Autodesk Inventor part; units mm, degrees
ref_plane "YZ Plane" through (0, 0, 0) normal (1, 0, 0) x (0, 1, 0)
ref_plane "XZ Plane" through (0, 0, 0) normal (0, 1, 0) x (-1, 0, 0)
ref_plane "XY Plane" through (0, 0, 0) normal (0, 0, 1) x (1, 0, 0)
sketch "Sketch1" plane through (0, 0, 0) normal (1, 0, 0) x (0, 1, 0)
  line L0 (0, 0) -> (15.2005, 26.3281)
  line L1 (15.2005, 26.3281) -> (43.7967, 9.8181)
  line L2 (0, -98.8011) -> (0, 41.6267)
  line L3 (43.7967, 9.8181) -> (0, -66.04)
  line L4 (0, 0) -> (0, -66.04)
  line L5 (19.05, 24.1056) -> (0, -8.89) construction
  dimension "d0" = 33.02
  dimension "d1" = 30
  dimension "d5" = 4.445
  dimension "d6" = 38.1
extrude "Extrusion1" add sketch "Sketch1" along normal mid plane 33.02
sketch "Sketch2" plane through (-16.51, 15.2005, 26.3281) normal (0, 0.5, 0.8660254) x (1, 0, 0)
  line L0 (0, 0) -> (33.02, 0) construction
  line L1 (33.02, 0) -> (33.02, 33.02) construction
  line L2 (0, 0) -> (33.02, 33.02) construction
  line L3 (33.02, 33.02) -> (0, 33.02) construction
  line L4 (0, 33.02) -> (33.02, 0) construction
  line L5 (3.175, 3.175) -> (29.845, 3.175)
  line L6 (29.845, 3.175) -> (29.845, 29.845)
  line L7 (29.845, 29.845) -> (3.175, 29.845)
  line L8 (3.175, 29.845) -> (3.175, 3.175)
  line L9 (3.175, 3.175) -> (29.845, 29.845) construction
  line L10 (29.845, 3.175) -> (3.175, 29.845) construction
  point P0 (16.51, 0)
  point P1 (16.51, 16.51)
  dimension "d7" = 26.67
extrude "Extrusion2" cut sketch "Sketch2" against normal blind 38.1
sketch "Sketch3" plane through (0, 0, 0) normal (1, 0, 0) x (0, 1, 0)
  line L0 (15.2005, 26.3281) -> (0, 0)
  line L1 (0, 0) -> (0, -66.04)
  line L2 (0, -66.04) -> (43.7967, 9.8181)
  line L3 (21.997, -21.59) -> (0, -8.89)
  line L4 (17.9501, 24.7406) -> (0, -6.35)
  line L5 (0, 0) -> (0, -66.04)
  line L6 (15.2005, 26.3281) -> (1.6498, 26.3281) construction
  line L7 (0, 0) -> (15.2005, 26.3281)
  line L8 (0, 0) -> (0, 51.7281)
  line L9 (43.7967, 9.8181) -> (0, -66.04)
  line L10 (0, -66.04) -> (0, -91.44)
  line L11 (0, -134.3611) -> (0, 77.1867)
  line L12 (0, 51.7281) -> (-3.175, 51.7281)
  line L13 (-3.175, 51.7281) -> (-3.175, -91.44)
  line L14 (-3.175, -91.44) -> (0, -91.44)
  point P0 (1.0999, -13.335)
  point P1 (0, -15.24)
  point P2 (0, -6.35)
  dimension "d10" = 25.4
  dimension "d11" = 25.4
  dimension "d12" = 3.175
  dimension "supportBaseLength" = 143.1681
extrude "Extrusion3" add sketch "Sketch3" along normal mid plane 22.86
sketch "Sketch5" plane through (0, 0, 0) normal (1, 0, 0) x (0, 1, 0)
  line L0 (0, 0) -> (15.2005, 26.3281)
  line L1 (0, 51.7281) -> (0, 0)
  line L2 (15.2005, 26.3281) -> (43.7967, 9.8181)
  line L3 (15.2005, 26.3281) -> (0, 26.3281)
  line L4 (0, 0) -> (15.2005, 26.3281)
extrude "Extrusion5" add sketch "Sketch5" along normal mid plane 22.86
sketch "Sketch4" plane through (0, 0, 0) normal (0, 0, 1) x (1, 0, 0)
  line L0 (16.51, 43.7967) -> (-16.51, 43.7967)
  line L1 (16.51, 0) -> (16.51, 43.7967)
  line L2 (16.51, 0) -> (11.43, 0)
  line L3 (11.43, 0) -> (-11.43, 0)
  line L4 (-11.43, 0) -> (-16.51, 0)
  line L5 (-16.51, 43.7967) -> (-16.51, 0)
  line L6 (-11.43, 0) -> (-11.43, -3.175)
  line L7 (11.43, -3.175) -> (-11.43, -3.175)
  line L8 (11.43, -3.175) -> (11.43, 0)
  line L9 (-11.43, 0) -> (-16.51, 5.08)
  line L10 (-16.51, 43.7967) -> (-16.51, 0)
  line L11 (-16.51, 5.08) -> (-16.51, 0)
  line L12 (0, 0) -> (0, 43.7967) construction
  line L13 (11.43, 0) -> (16.51, 0)
  line L14 (11.43, 0) -> (16.51, 5.08)
  line L15 (16.51, 5.08) -> (16.51, 0)
  dimension "d15" = 45
extrude "Extrusion4" cut sketch "Sketch4" against normal up to surface (143.1681 mm away) from surface at 51.7281 contours L1 L2 L14 | L9 L4 L5
sketch "Sketch6" plane through (-11.43, 0, 51.7281) normal (0, 1, 0) x (1, 0, 0)
  line L0 (22.86, 143.1681) -> (0, 143.1681) construction
  line L1 (11.43, 143.1681) -> (11.43, 0) construction
  line L2 (22.86, 0) -> (0, 0) construction
  point P0 (11.43, 51.7281)
  point P1 (11.43, 130.4681)
  point P2 (11.43, 12.7)
  dimension "d21" = 12.7
  dimension "d22" = 12.7
hole "Hole1" at (0, 0, -78.74) at (0, 0, 39.0281) direction (0, -1, 0) diameter 5.6134 end through all
sketch "Sketch9" plane through (0, 0, 0) normal (1, 0, 0) x (0, 1, 0)
  line L0 (1.905, -3.0504) -> (1.905, -9.9899)
  line L1 (1.905, -9.9899) -> (21.997, -21.59)
  line L2 (41.047, 11.4056) -> (21.997, -21.59)
  line L3 (17.9501, 24.7406) -> (41.047, 11.4056)
  line L4 (17.9501, 24.7406) -> (1.905, -3.0504)
  line L5 (29.4986, 18.0731) -> (10.4486, -14.9225) construction
  line L6 (1.905, -9.9899) -> (21.997, -21.59) construction
  circle A0 centre (19.9736, 1.5753) radius 2.8067
  point P0 (0, 0)
  dimension "d30" = 5.6134
extrude "Extrusion6" cut sketch "Sketch9" along normal through all both and the other way through all contours A0
sketch "Sketch10" plane through (-16.51, 43.7967, 9.8181) normal (0, 0.8660254, -0.5) x (1, 0, 0)
  line L0 (3.175, 0) -> (29.845, 0) construction
  line L1 (16.51, 0) -> (16.51, 77.7875) construction
  point P0 (16.51, 30.401)
  point P1 (16.51, 19.05)
  dimension "d33" = 19.05
hole "Hole2" at (0, 34.2717, -6.6797) direction (0, -0.8660254, 0.5) diameter 5.6134 depth 3.175
equation "\"d0\" = widthToSupportExtrusion"
equation "\"d1\" = attachementAngle"
equation "\"d6\" = insertDepth"
equation "\"d2\" = widthToSupportExtrusion"
equation "\"d7\" = insertForExtrusion"
equation "\"d8\" = insertDepth"
equation "\"d12\" = supportBaseDepth"
equation "\"d13\" = supportBaseWidth"
equation "\"attachementAngle\" = 30deg"
equation "\"extrusionSize\" = 25.4"
equation "\"wallThickness\" = 3.175"
equation "\"slipClearance\" = 0.635"
equation "\"insertForExtrusion\" = extrusionSize + 2 * slipClearance"
equation "\"widthToSupportExtrusion\" = insertForExtrusion + 2 * wallThickness"
equation "\"insertDepth\" = 38.1"
equation "\"supportBaseWidth\" = 22.86"
equation "\"supportBaseDepth\" = 3.175"
properties part number "30DegreeAttachementV04"
Verification items for the finished model (mm, model axes). A direction names the side the tool comes from. Coordinates: 2 decimals unless noted, no trailing zeros. Order: outer loops, then holes, each group sorted by start corner. A loop starts at its lowest first (then second) coordinate and runs counter-clockwise, first axis right, second up. Notation, with made-up numbers: M 40.25,-35 L 70.25,-35 A21 cw 70.25,-21 Z; hole C 84.5,-2.75 d11. An arc over 180 degrees is marked long. Return JSON: item names as keys, results as strings.
1) Cross-section at D-D, the plane x = 9.5. Record the boundary of the cut face in (y, z) (1 decimal), and give its area (3 significant figures).
Answer list:
{"outline": "M -3.2,-91.4 L 0,-91.4 L 0,-66 L 43.8,9.8 L 41,11.4 L 22,-21.6 L 0,-8.9 L 0,-6.3 L 18,24.7 L 15.2,26.3 L 0,26.3 L 0,51.7 L -3.2,51.7 Z", "area": "1,590 mm2"}
2) Cross-section at B-B, the plane x = 1.5. Record the boundary of the cut face in (y, z) (1 decimal).
Answer list:
{"outline": "M -3.2,-91.4 L 0,-91.4 L 0,-81.1 L -3.2,-81.1 Z; M -3.2,-76.4 L 0,-76.4 L 0,-66 L 33.1,-8.7 L 30.3,-7.1 L 22,-21.6 L 0,-8.9 L 0,-6.3 L 18,24.7 L 15.2,26.3 L 0,26.3 L 0,36.7 L -3.2,36.7 Z; M -3.2,41.4 L 0,41.4 L 0,51.7 L -3.2,51.7 Z; M 32.7,-3 L 35.5,-4.6 L 43.8,9.8 L 41,11.4 Z"}
3) Cross-section at C-C, the plane y = 6.5. Record the boundary of the cut face in (x, z) (3 decimals), and give its area (3 significant figures).
Answer list:
{"outline": "M -16.51,-54.782 L 16.51,-54.782 L 16.51,11.258 L 11.43,11.258 L 11.43,26.328 L -11.43,26.328 L -11.43,11.258 L -16.51,11.258 Z; hole M -13.335,-12.645 L 13.335,-12.645 L 13.335,4.908 L -13.335,4.908 Z", "area": "2,060 mm2"}
4) Gauge pin test, flat ends, axial feed: pin 1 (1.5 mm diameter, centred on x = -4, y = 8, fed in from -Z); pin 2 (11.5 mm diameter, centred on x = -1, z = 35, fed in from +Y); pin 3 (4.5 mm diameter, centred on y = 19.97, z = 1.58, fed in from -X); pin 4 (5 mm diameter, centred on x = 12.5, y = 32.5, fed in from +Z). Record the tip position at first contact, or that the pin passes through.
Answer list:
{"pin 1": "z = -53.48", "pin 2": "y = 0", "pin 3": "through", "pin 4": "z = 17.7"}
5) Cross-section at A-A, the plane z = -78.74. Record the boundary of the cut face in (x, y) (3 decimals).
Answer list:
{"outline": "M -11.43,-3.175 L -2.807,-3.175 L -2.807,0 L -11.43,0 Z; M 2.807,-3.175 L 11.43,-3.175 L 11.43,0 L 2.807,0 Z"}
6) Release check for a two-part mould opening along Z. For faces 1 (the flat face through (-0.2, 0, -75.7)), 2 (the cylindrical face through (-0.123, 31.476, -8.303)), 3 (the flat face through (0, 8, 26.328)), 4 (the flat face through (-0.19, 9.1, 9.41)) record: +Z half, -Z half, draft (parallel to the pull), parting line (faces both ways), or undercut.
Answer list:
{"face 1": "draft", "face 2": "undercut", "face 3": "+Z half", "face 4": "undercut"}
7) Access from +Z, -Z, +X, -X, +Y, -Y to the whole of each face (thin tool, end or side, straight path). Record for faces 5 (the flat face through (-14.006, 9.183, 15.905)), 6 (the flat face through (13.934, 9.183, 15.905)), 7 (the flat face through (0, 0, 42)).
Answer list:
{"face 5": "+Z, -X, -Y", "face 6": "+Z, +X, -Y", "face 7": "+Z, +X, -X, +Y"}
8) Thickness scan on L1, parallel to Z at x = 0, y = -1.55; L2, parallel to X at y = 15.5, z = 1.5 (3 decimals); L3, parallel to Y at x = -1, z = -16.5 (3 decimals). Record the ranges inside material, lowest first. Write a range as [from, to].
Answer list:
{"L1": "[-91.44, -81.55], [-75.93, 36.22], [41.83, 51.73]", "L2": "[-16.51, -13.335], [13.335, 16.51]", "L3": "[-3.175, 13.177], [24.936, 28.602]"}
